```python
from build123d import *

# Parameters (mm, degrees)
BASE_FLANGE1_DEPTH           = 1.5
EDGE_FLANGE1_STRIP_W         = 7.4732
EDGE_FLANGE1_STRIP_H         = 1.5
EDGE_FLANGE1_STRIP_CUT_DEPTH = 10
EDGE_FLANGE1_DEPTH           = 10
M3_TAPPED_HOLE1_D            = 2.5
M3_TAPPED_HOLE1_CSINK_D      = 3.05
M3_TAPPED_HOLE1_CSINK_ANGLE  = 90
MIRROR2_COPY_1_SKETCH_W      = 7.4732
MIRROR2_COPY_1_SKETCH_H      = 1.5
MIRROR2_COPY_1_DEPTH         = 10
MIRROR2_COPY_2_DEPTH         = 10
MIRROR2_COPY_3_D             = 2.5
MIRROR2_COPY_3_CSINK_D       = 3.05
MIRROR2_COPY_3_CSINK_ANGLE   = 90
M4_TAPPED_HOLE1_D            = 3.3
M4_TAPPED_HOLE1_CSINK_D      = 4.05
M4_TAPPED_HOLE1_CSINK_ANGLE  = 90


# Sheet-metal steps are written as plain solids
with BuildPart() as part:
    # Sketch1 → Base-Flange1 (new body)
    with BuildSketch(Plane(origin=(0, 0, 0), x_dir=(1, 0, 0), z_dir=(0, 1, 0))):
        Polygon((-41, -34.62), (-41, -49), (41, -49), (41, -34.62), (50, -34.62), (50, -24.62), (41, -24.62), (41, 24.62), (50, 24.62), (50, 34.62), (41, 34.62), (41, 49), (-41, 49), (-41, 34.62), (-50, 34.62), (-50, 24.62), (-41, 24.62), (-41, -24.62), (-50, -24.62), (-50, -34.62), align=None)
    extrude(amount=-BASE_FLANGE1_DEPTH)

    # Edge-Flange1 strip (across the edge) → Edge-Flange1 strip cut (cut)
    with BuildSketch(Plane(origin=(-50, -1.5, 34.62), x_dir=(1, 0, 0), z_dir=(0, 0, -1))):
        with Locations((-1.5, -0.75)):
            Rectangle(EDGE_FLANGE1_STRIP_W, EDGE_FLANGE1_STRIP_H)
    edge_flange1_strip_cut = extrude(amount=EDGE_FLANGE1_STRIP_CUT_DEPTH, mode=Mode.SUBTRACT)

    # Edge-Flange1 section (across the edge) → Edge-Flange1 (add)
    with BuildSketch(Plane(origin=(-50, -1.5, 34.62), x_dir=(1, 0, 0), z_dir=(0, 0, -1))):
        with BuildLine():
            Line((0, 0.7366), (0, 25.5))
            Line((0, 25.5), (1.5, 25.5))
            Line((1.5, 25.5), (1.5, 0.7366))
            ThreePointArc((1.5, 0.7366), (1.715745145, 0.215745145), (2.2366, 0))
            Line((2.2366, 0), (2.2366, -1.5))
            ThreePointArc((2.2366, -1.5), (0.655084973, -0.844915027), (0, 0.7366))
        make_face()
    edge_flange1 = extrude(amount=EDGE_FLANGE1_DEPTH)

    # M3 Tapped Hole1 (through all)
    with Locations(Plane.ZY.offset(50)):
        with Locations((29.62, -8), (29.62, -23)):
            m3_tapped_hole1 = CounterSinkHole(M3_TAPPED_HOLE1_D / 2, M3_TAPPED_HOLE1_CSINK_D / 2, counter_sink_angle=M3_TAPPED_HOLE1_CSINK_ANGLE)

    # Mirror1: Edge-Flange1 strip cut, Edge-Flange1, M3 Tapped Hole1 across plane
    add(edge_flange1_strip_cut.mirror(Plane(origin=(0, 0, 0), x_dir=(0, 0, 1), z_dir=(1, 0, 0))), mode=Mode.SUBTRACT)
    add(edge_flange1.mirror(Plane(origin=(0, 0, 0), x_dir=(0, 0, 1), z_dir=(1, 0, 0))))
    add(m3_tapped_hole1.mirror(Plane(origin=(0, 0, 0), x_dir=(0, 0, 1), z_dir=(1, 0, 0))), mode=Mode.SUBTRACT)

    # Mirror2: Edge-Flange1 strip cut, Edge-Flange1, M3 Tapped Hole1 across plane
    add(edge_flange1_strip_cut.mirror(Plane.XY), mode=Mode.SUBTRACT)
    add(edge_flange1.mirror(Plane.XY))
    add(m3_tapped_hole1.mirror(Plane.XY), mode=Mode.SUBTRACT)

    # Mirror2 copy 1 sketch → Mirror2 copy 1 (cut)
    with BuildSketch(Plane(origin=(50, -1.5, -34.62), x_dir=(-1, 0, 0), z_dir=(0, 0, 1))):
        with Locations((-1.5, -0.75)):
            Rectangle(MIRROR2_COPY_1_SKETCH_W, MIRROR2_COPY_1_SKETCH_H)
    extrude(amount=MIRROR2_COPY_1_DEPTH, mode=Mode.SUBTRACT)

    # Mirror2 copy 2 sketch → Mirror2 copy 2 (add)
    with BuildSketch(Plane(origin=(50, -1.5, -34.62), x_dir=(-1, 0, 0), z_dir=(0, 0, 1))):
        with BuildLine():
            Line((0, 0.7366), (0, 25.5))
            Line((0, 25.5), (1.5, 25.5))
            Line((1.5, 25.5), (1.5, 0.7366))
            ThreePointArc((1.5, 0.7366), (1.715745145, 0.215745145), (2.2366, 0))
            Line((2.2366, 0), (2.2366, -1.5))
            ThreePointArc((2.2366, -1.5), (0.655084973, -0.844915027), (0, 0.7366))
        make_face()
    extrude(amount=MIRROR2_COPY_2_DEPTH)

    # Mirror2 copy 3 (through all)
    with Locations(Plane(origin=(50, 0, 0), x_dir=(0, 0, -1), z_dir=(1, 0, 0))):
        with Locations((29.62, -8), (29.62, -23)):
            CounterSinkHole(MIRROR2_COPY_3_D / 2, MIRROR2_COPY_3_CSINK_D / 2, counter_sink_angle=MIRROR2_COPY_3_CSINK_ANGLE)

    # M4 Tapped Hole1 (through all)
    with Locations(Plane(origin=(0, 0, 0), x_dir=(1, 0, 0), z_dir=(0, 1, 0))):
        with Locations((-32, 29.62), (0, 29.62), (32, 29.62), (-32, -29.62), (0, -29.62), (32, -29.62), (0, 43.62), (0, -43.62)):
            CounterSinkHole(M4_TAPPED_HOLE1_D / 2, M4_TAPPED_HOLE1_CSINK_D / 2, counter_sink_angle=M4_TAPPED_HOLE1_CSINK_ANGLE)


solid = part.part
```
Geometry: final body of the model. Coordinates: model frame, mm. A direction names the side the tool comes from. Coordinates: 2 decimals unless noted, no trailing zeros. Write each loop counter-clockwise with the first axis right and the second up, starting at its lowest first coordinate (ties: lowest second). Pieces come first, ordered by that corner, then holes. Notation, with made-up numbers: M 23.5,-24.5 L 54.5,-24.5 A21 ccw 54.5,5.5 Z; hole C -21.75,77.5 d4. An arc over 180 degrees is marked long. Answer as CSV lines item,"result". Start each with the question number.
Q1. Mould query, pull axis Y, two halves, no side actions, for faces 4 (the cylindrical face through (49.33, -0.64, 29.69)), 5 (the cylindrical face through (-49.104, -24.109, -29.043)), 6 (the cylindrical face through (-49.104, -8.479, 28.465)), 7 (the cylindrical face through (0.215, -0.945, 27.984)). Classes: released by +Y, released by -Y, zero draft, split by the parting line, or undercut.
Q2. Pin query (flat end, axial travel): P1, Ø2.5, axis at x = -47.5, y = -17.5, coming from the -Z side; P2, Ø2.5, axis at x = 0, z = 43.62, coming from the +Y side; P3, Ø1.6, axis at y = -0.5, z = 3, coming from the -X side; P4, Ø10, axis at x = 45.5, y = -7, coming from the +Z side. Return the tip coordinate at first contact, or that it passes through.
Q3. Line query: line 1 (Y direction, x = 49, z = 29.62); line 2 (Z direction, x = -49.2, y = -8); line 3 (Z direction, x = -32, y = -1.2). Output: solid intervals per line, ascending. Write a range as from..to.
Q4. Cut plane A-A on x = -32. Return the cut outline in (y, z) (3 decimals).
Q5. Cut plane B-B on z = 43.62. Return the cut outline in (x, y) (3 decimals).
Q6. Cut plane C-C on x = 0. Return the cut outline in (y, z) (3 decimals).
Q7. Cut plane D-D on y = -16.75. Return the cut outline in (x, z).
Q8. Reachability of faces 1 (the flat face through (49, -12, -34.62)), 2 (the flat face through (-48.5, -15, 30)), 3 (the cylindrical face through (-30.35, -0.95, -29.69)) from +Z, -Z, +X, -X, +Y, -Y: full face, straight path, thin tool, end or side. Return the list, or none.
Findings below:
1,face 4,"released by +Y"
1,face 5,"undercut"
1,face 6,"undercut"
1,face 7,"zero draft"
2,P1,"stops at z = -34.62"
2,P2,"passes through"
2,P3,"stops at x = -41"
2,P4,"stops at z = 34.62"
3,line 1,"y = -27..-24.25, -21.75..-9.25, -6.75..-0.37"
3,line 2,"z = -34.62..-30.87, -28.37..-24.62, 24.62..28.37, 30.87..34.62"
3,line 3,"z = -49..-31.27, -27.97..27.97, 31.27..49"
4,outline,"M -1.5,-49 L 0,-49 L 0,-31.645 L -0.375,-31.27 L -1.5,-31.27 Z; M -1.5,-27.97 L -0.375,-27.97 L 0,-27.595 L 0,27.595 L -0.375,27.97 L -1.5,27.97 Z; M -1.5,31.27 L -0.375,31.27 L 0,31.645 L 0,49 L -1.5,49 Z"
5,outline,"M -41,-1.5 L -1.65,-1.5 L -1.65,-0.375 L -2.025,0 L -41,0 Z; M 1.65,-1.5 L 41,-1.5 L 41,0 L 2.025,0 L 1.65,-0.375 Z"
6,outline,"M -1.5,-49 L 0,-49 L 0,-45.645 L -0.375,-45.27 L -1.5,-45.27 Z; M -1.5,-41.97 L -0.375,-41.97 L 0,-41.595 L 0,-31.645 L -0.375,-31.27 L -1.5,-31.27 Z; M -1.5,-27.97 L -0.375,-27.97 L 0,-27.595 L 0,27.595 L -0.375,27.97 L -1.5,27.97 Z; M -1.5,31.27 L -0.375,31.27 L 0,31.645 L 0,41.595 L -0.375,41.97 L -1.5,41.97 Z; M -1.5,45.27 L -0.375,45.27 L 0,45.645 L 0,49 L -1.5,49 Z"
7,outline,"M -50,-34.62 L -48.5,-34.62 L -48.5,-24.62 L -50,-24.62 Z; M -50,24.62 L -48.5,24.62 L -48.5,34.62 L -50,34.62 Z; M 48.5,-34.62 L 50,-34.62 L 50,-24.62 L 48.5,-24.62 Z; M 48.5,24.62 L 50,24.62 L 50,34.62 L 48.5,34.62 Z"
8,face 1,"-Z, +X, +Y, -Y"
8,face 2,"+Z, -Z, -Y"
8,face 3,"+Y, -Y"
